Read the model definition and answer for the solid it produces. Units are mm, in the model's axes. A direction names the side the tool comes from. Give positions to 0.01 mm unless a question says otherwise; leave off trailing zeros. Loops run counter-clockwise (first coordinate to the right, second up) from the corner with the lowest first, then second, coordinate; pieces in that order, holes last. Notation, with made-up numbers: (60, -22) - (99, -22) arc R23 cw to (99, 13) - close; hole circle Ø5 at (80.5, -9). An arc over 180 degrees is marked (long way). Write each question's results on one line, items separated by ' | '. Start each with the question number.
Q1. The part is cut by section C-C, the plane x = 3.5. Write down the section's boundary in (y, z).
Q2. Find the intervals of material crossed by line 1 (Y direction, x = 3.15, z = 0); line 2 (Y direction, x = 1.45, z = 0); line 3 (Z direction, x = 1, y = 5), in increasing order. Write a range as from..to.
Q3. Determine the mould class of faces 1 (the cylindrical face through (2.64, -7.84, 5)), 2 (the cylindrical face through (3.5, -3.2, 10)), 3 (the flat face through (0, 9, -4)) for opening direction Z: +Z half, -Z half, draft (parallel to the pull), parting line (faces both ways), or undercut.
Q4. Given pin 1 (3 mm diameter, centred on y = -4, z = -0.5, fed in from -X); pin 2 (2 mm diameter, centred on y = -5, z = 4, fed in from -X); pin 3 (4 mm diameter, centred on x = 6, y = 8, fed in from -Z), each flat-ended and moving along its own axis, determine where each tip first touches the part or whether it passes through.
Q5. For faces 4 (the cylindrical face through (3.7, -2.16, 6.87)), 5 (the cylindrical face through (3.549, -1.802, 5.723)), 6 (the cylindrical face through (0.37, -2.16, 6.87)), determine the directions among +Z, -Z, +X, -X, +Y, -Y from which every point of the face is accessible in a straight line to the end or side of a thin tool.
Q6. The part is cut by section A-A, the plane z = 0. Write down the section's boundary in (x, y), plus the area to 3 significant figures.
```python
from build123d import *

# Parameters (mm, degrees)
SKETCH_2_R = 0.75
FILLET_1_R = 0.3


with BuildPart() as part:
    # 草图2 → 旋转1 (revolve)
    with BuildSketch(Plane.XY, mode=Mode.PRIVATE) as revolve_1_sk:
        with BuildLine():
            ThreePointArc((2.25, 7.2), (1.5, 7.95), (0.75, 7.2))
            Line((0.75, 7.2), (2.25, 7.2))
        make_face()
        with BuildLine():
            Line((2.25, 7.2), (0.75, 7.2))
            ThreePointArc((0.75, 7.2), (1.5, 6.45), (2.25, 7.2))
        make_face()
        with Locations((1.5, 7.2)):
            Circle(SKETCH_2_R)
        Polygon((5.5, 7.2), (0, 7.2), (0, 6), (7, 6), (7, 10.5), (0, 10.5), (0, 9.3), (5.5, 9.3), align=None)
    revolve(revolve_1_sk.sketch.rotate(Axis((-18.653285905, 0, 0), (1, 0, 0)), 90), axis=Axis((-18.653285905, 0, 0), (1, 0, 0)))

    # 圆角1
    fillet_1_edges = [part.edges().sort_by_distance(p)[0] for p in [
        (5.5, 0, -7.2),
        (5.5, 0, -9.3),
    ]]
    fillet(fillet_1_edges, radius=FILLET_1_R)


solid = part.part
```
Check sheet entries:
1) outline: circle Ø21 at (0, 0); circle Ø14.4 at (0, 0); hole circle Ø18.6 at (0, 0); hole circle Ø12 at (0, 0)
2) line 1: y = -10.5..-9.3, -7.2..-6, 6..7.2, 9.3..10.5 | line 2: y = -10.5..-9.3, -7.95..-6, 6..7.95, 9.3..10.5 | line 3: z = -9.23..-7.84, -5.93..-3.32, 3.32..5.93, 7.84..9.23
3) face 1: undercut | face 2: parting line | face 3: draft
4) pin 1: passes through | pin 2: stops at x = 0 | pin 3: stops at z = -8.62
5) face 4: none | face 5: +X, -X | face 6: -X
6) outline: (0, -10.5) - (7, -10.5) - (7, -6) - (0, -6) - (0, -7.2) - (0.75, -7.2) arc R0.75 ccw to (2.25, -7.2) - (5.2, -7.2) arc R0.3 cw to (5.5, -7.5) - (5.5, -9) arc R0.3 cw to (5.2, -9.3) - (0, -9.3) - close; (0, 6) - (7, 6) - (7, 10.5) - (0, 10.5) - (0, 9.3) - (5.2, 9.3) arc R0.3 cw to (5.5, 9) - (5.5, 7.5) arc R0.3 cw to (5.2, 7.2) - (2.25, 7.2) arc R0.75 ccw to (0.75, 7.2) - (0, 7.2) - close | area: 41.7 mm^2
